Geometry check sheet. Reference: the model listing, model coordinates, mm. Face numbers are marked on the shaded views. A direction names the side the tool comes from. Round coordinates to 2 decimals unless told otherwise and drop trailing zeros. Write each loop counter-clockwise with the first axis right and the second up, starting at its lowest first coordinate (ties: lowest second). Pieces come first, ordered by that corner, then holes. Notation, with made-up numbers: M 1,-26.75 L 59,-26.75 A18 ccw 59,2.25 Z; hole C -14.5,31.5 d5. An arc over 180 degrees is marked long. Use a Markdown table: item, result.
```python
from build123d import *

# Parameters (mm, degrees)
EXTRUDE_1_DEPTH               = 9
CUT_EXTRUDE_1_DEPTH           = 30.816103032
CUT_EXTRUDE_1_DEPTH_BACK      = 30.816103032
SKETCH_2_R                    = 2.3
CUT_EXTRUDE_2_DEPTH           = 3.3
CUT_EXTRUDE_2_OTHER_WAY_DEPTH = 36.043722716
CUT_EXTRUDE_2_OTHER_WAY_TAPER = 1
CUT_EXTRUDE_3_DEPTH           = 36.043722716
CUT_EXTRUDE_3_DEPTH_BACK      = 4
CUT_EXTRUDE_4_REACH           = 46.777
CUT_EXTRUDE_4_END_RADIUS      = 10.2
SKETCH_5_R                    = 1.6
EXTRUDE_2_DEPTH               = 3
SKETCH_7_W                    = 6.2
SKETCH_7_H                    = 6
CUT_EXTRUDE_6_DEPTH           = 1
CHAMFER_3_SIZE                = 1
CUT_EXTRUDE_8_REACH           = 35.645
SKETCH_9_R                    = 2.2
CUT_EXTRUDE_9_DEPTH           = 30.816103122
CUT_EXTRUDE_START             = 5.5
SKETCH_10_R                   = 4
SKETCH_10_R_2                 = 2.2
CUT_EXTRUDE_10_DEPTH          = 5.5


with BuildPart() as part:
    # Эскиз1 → Бобышка-Вытянуть1 (new, symmetric)
    with BuildSketch(Plane(origin=(0, 0, 0), x_dir=(0, 0, -1), z_dir=(1, 0, 0))):
        with BuildLine():
            Line((-0.75, -21), (-0.75, -11.06243644))
            ThreePointArc((-0.75, -11.06243644), (-0.989654684, -10.412917388), (-1.59375, -10.074718901))
            ThreePointArc((-1.59375, -10.074718901), (0, 10.2), (1.59375, -10.074718901))
            ThreePointArc((1.59375, -10.074718901), (0.989654684, -10.412917388), (0.75, -11.06243644))
            Line((0.75, -11.06243644), (0.75, -21))
            ThreePointArc((0.75, -21), (1.042893219, -21.707106781), (1.75, -22))
            Line((1.75, -22), (6.75, -22))
            ThreePointArc((6.75, -22), (7.457106781, -21.707106781), (7.75, -21))
            Line((7.75, -21), (7.75, -13.898830886))
            ThreePointArc((7.75, -13.898830886), (8.121662204, -12.215036114), (9.167582418, -10.844142779))
            ThreePointArc((9.167582418, -10.844142779), (13.897042702, -2.917568189), (12.75462481, 6.241758242))
            ThreePointArc((12.75462481, 6.241758242), (12.953882386, 10.117431577), (16.34747687, 12))
            Line((16.34747687, 12), (17, 12))
            ThreePointArc((17, 12), (17.707106781, 12.292893219), (18, 13))
            Line((18, 13), (18, 18))
            Line((18, 18), (-18, 18))
            Line((-18, 18), (-18, 13))
            ThreePointArc((-18, 13), (-17.707106781, 12.292893219), (-17, 12))
            Line((-17, 12), (-16.34747687, 12))
            ThreePointArc((-16.34747687, 12), (-12.953882386, 10.117431577), (-12.75462481, 6.241758242))
            ThreePointArc((-12.75462481, 6.241758242), (-13.897042702, -2.917568189), (-9.167582418, -10.844142779))
            ThreePointArc((-9.167582418, -10.844142779), (-8.121662204, -12.215036114), (-7.75, -13.898830886))
            Line((-7.75, -13.898830886), (-7.75, -21))
            ThreePointArc((-7.75, -21), (-7.457106781, -21.707106781), (-6.75, -22))
            Line((-6.75, -22), (-1.75, -22))
            ThreePointArc((-1.75, -22), (-1.042893219, -21.707106781), (-0.75, -21))
        make_face()
    extrude(amount=EXTRUDE_1_DEPTH, both=True)

    # Эскиз2 → Вырез-Вытянуть1 (cut, two sides: drawn at the far end of the back side and taken through both)
    with BuildSketch(Plane.XY.offset(-CUT_EXTRUDE_1_DEPTH_BACK)):
        with BuildLine():
            ThreePointArc((-3.1, 18), (0, 14.9), (3.1, 18))
            Line((3.1, 18), (-3.1, 18))
        make_face()
        with Locations(Location((0, -16, 0), (0, 0, 66.000891847))):
            Circle(SKETCH_2_R)
    extrude(amount=CUT_EXTRUDE_1_DEPTH + CUT_EXTRUDE_1_DEPTH_BACK, mode=Mode.SUBTRACT)

    # Эскиз3 → Вырез-Вытянуть2 (cut)
    with BuildSketch(Plane(origin=(0, 0, -7.75), x_dir=(-1, 0, 0), z_dir=(0, 0, -1))):
        Polygon((-4.618802154, -16), (-2.309401077, -20), (2.309401077, -20), (4.618802154, -16), (2.309401077, -12), (-2.309401077, -12), align=None)
    extrude(amount=-CUT_EXTRUDE_2_DEPTH, mode=Mode.SUBTRACT)

    # Эскиз3 → Вырез-Вытянуть2 other way (cut)
    with BuildSketch(Plane(origin=(0, 0, -7.75), x_dir=(-1, 0, 0), z_dir=(0, 0, -1))):
        Polygon((-4.618802154, -16), (-2.309401077, -20), (2.309401077, -20), (4.618802154, -16), (2.309401077, -12), (-2.309401077, -12), align=None)
    extrude(amount=CUT_EXTRUDE_2_OTHER_WAY_DEPTH, taper=CUT_EXTRUDE_2_OTHER_WAY_TAPER, mode=Mode.SUBTRACT)

    # Эскиз4 → Вырез-Вытянуть3 (cut, two sides: drawn at the far end of the back side and taken through both)
    with BuildSketch(Plane.XY.offset(7.75).offset(-CUT_EXTRUDE_3_DEPTH_BACK)):
        with BuildLine():
            Line((-3.403687464, -13.898830886), (-0.935461573, -13.898830886))
            ThreePointArc((-0.935461573, -13.898830886), (0, -18.3), (0.935461573, -13.898830886))
            Line((0.935461573, -13.898830886), (3.403687464, -13.898830886))
            ThreePointArc((3.403687464, -13.898830886), (0, -12), (-3.403687464, -13.898830886))
        make_face()
        with BuildLine():
            ThreePointArc((0.935461573, -13.898830886), (0, -18.3), (-0.935461573, -13.898830886))
            Line((-0.935461573, -13.898830886), (-3.403687464, -13.898830886))
            ThreePointArc((-3.403687464, -13.898830886), (-1.092073748, -19.848035204), (4, -16))
            ThreePointArc((4, -16), (3.848035204, -14.907926252), (3.403687464, -13.898830886))
            Line((3.403687464, -13.898830886), (0.935461573, -13.898830886))
        make_face()
        with BuildLine():
            Line((-3.403687464, -13.898830886), (-0.935461573, -13.898830886))
            ThreePointArc((-0.935461573, -13.898830886), (0, -18.3), (0.935461573, -13.898830886))
            Line((0.935461573, -13.898830886), (3.403687464, -13.898830886))
            ThreePointArc((3.403687464, -13.898830886), (0, -12), (-3.403687464, -13.898830886))
        make_face()
        with BuildLine():
            ThreePointArc((0.935461573, -13.898830886), (0, -18.3), (-0.935461573, -13.898830886))
            Line((-0.935461573, -13.898830886), (-3.403687464, -13.898830886))
            ThreePointArc((-3.403687464, -13.898830886), (-1.092073748, -19.848035204), (4, -16))
            ThreePointArc((4, -16), (3.848035204, -14.907926252), (3.403687464, -13.898830886))
            Line((3.403687464, -13.898830886), (0.935461573, -13.898830886))
        make_face()
    extrude(amount=CUT_EXTRUDE_3_DEPTH + CUT_EXTRUDE_3_DEPTH_BACK, mode=Mode.SUBTRACT)

    # Вырез-Вытянуть4: up to this cylinder (the profile starts outside it)
    cut_extrude_4_end = Plane(origin=(0, 0, 0), z_dir=(-1, 0, 0)) * Cylinder(CUT_EXTRUDE_4_END_RADIUS, 127.454, mode=Mode.PRIVATE)
    # Эскиз5 → Вырез-Вытянуть4 (cut, up to the surface)
    with BuildSketch(Plane(origin=(0, 18, 0), x_dir=(1, 0, 0), z_dir=(0, 1, 0)), mode=Mode.PRIVATE) as cut_extrude_4_sk1:
        with Locations(Location((6.25, 0, 0), (0, 0, 270))):
            Circle(SKETCH_5_R)
    cut_extrude_4_tool1 = extrude(cut_extrude_4_sk1.sketch, amount=-CUT_EXTRUDE_4_REACH, mode=Mode.PRIVATE) - cut_extrude_4_end
    add(cut_extrude_4_tool1.solids().sort_by_distance((6.25, 18, 0))[0], mode=Mode.SUBTRACT)
    # Эскиз5 → Вырез-Вытянуть4 (cut, up to the surface)
    with BuildSketch(Plane(origin=(0, 18, 0), x_dir=(1, 0, 0), z_dir=(0, 1, 0)), mode=Mode.PRIVATE) as cut_extrude_4_sk2:
        with Locations(Location((-6.25, 0, 0), (0, 0, 270))):
            Circle(SKETCH_5_R)
    cut_extrude_4_tool2 = extrude(cut_extrude_4_sk2.sketch, amount=-CUT_EXTRUDE_4_REACH, mode=Mode.PRIVATE) - cut_extrude_4_end
    add(cut_extrude_4_tool2.solids().sort_by_distance((-6.25, 18, 0))[0], mode=Mode.SUBTRACT)

    # Эскиз6 → Бобышка-Вытянуть2 (add, symmetric)
    with BuildSketch(Plane.XY):
        with BuildLine():
            Line((-3.1, 18), (3.1, 18))
            ThreePointArc((3.1, 18), (0, 14.9), (-3.1, 18))
        make_face()
    extrude(amount=EXTRUDE_2_DEPTH, both=True)

    # Эскиз7 → Вырез-Вытянуть6 (cut)
    with BuildSketch(Plane(origin=(0, 18, 0), x_dir=(1, 0, 0), z_dir=(0, 1, 0))):
        Rectangle(SKETCH_7_W, SKETCH_7_H)
    extrude(amount=-CUT_EXTRUDE_6_DEPTH, mode=Mode.SUBTRACT)

    # Фаска3
    # the kernel refuses this chamfer: 1 mm, written as the material it adds along each edge
    with BuildSketch(Plane(origin=(3.1, 17, -3), x_dir=(0.02749587661058651, 0.9996219169112968, 0), z_dir=(0, 0, 1))) as chamfer_3_piece_1_section:
        Polygon((CHAMFER_3_SIZE * 0.999621916911, CHAMFER_3_SIZE * 0.0274958766106), (-CHAMFER_3_SIZE * 0.0274958766106, CHAMFER_3_SIZE * 0.999621916911), (0, 0), align=None)
    chamfer_3_piece_1 = extrude(amount=6, mode=Mode.PRIVATE)
    chamfer_3_piece_1 = split(chamfer_3_piece_1, bisect_by=Plane(origin=(2.769595846, 18, 0), z_dir=(0, -1, 0)), keep=Keep.TOP, mode=Mode.PRIVATE)
    add(chamfer_3_piece_1)
    with BuildSketch(Plane(origin=(-3.1, 17, 3), x_dir=(-0.02749587661058651, 0.9996219169112968, 0), z_dir=(0, 0, -1))) as chamfer_3_piece_2_section:
        Polygon((CHAMFER_3_SIZE * 0.999621916911, CHAMFER_3_SIZE * 0.0274958766106), (-CHAMFER_3_SIZE * 0.0274958766106, CHAMFER_3_SIZE * 0.999621916911), (0, 0), align=None)
    chamfer_3_piece_2 = extrude(amount=6, mode=Mode.PRIVATE)
    chamfer_3_piece_2 = split(chamfer_3_piece_2, bisect_by=Plane(origin=(-2.769595846, 18, 0), z_dir=(0, -1, 0)), keep=Keep.TOP, mode=Mode.PRIVATE)
    add(chamfer_3_piece_2)

    # Вырез-Вытянуть8: up to this plane
    cut_extrude_8_end = Plane(origin=(3.1, 18, 0), z_dir=(-0.7071067811865525, 0.7071067811865426, 0))
    # Эскиз8 → Вырез-Вытянуть8 (cut, up to the surface)
    with BuildSketch(Plane(origin=(9, 0, 0), x_dir=(0, 0, -1), z_dir=(1, 0, 0)), mode=Mode.PRIVATE) as cut_extrude_8_sk1:
        with BuildLine():
            ThreePointArc((-10.25, 18), (-6.75, 14.5), (-3.25, 18))
            Line((-3.25, 18), (-10.25, 18))
        make_face()
    cut_extrude_8_tool1 = split(extrude(cut_extrude_8_sk1.sketch, amount=-CUT_EXTRUDE_8_REACH, mode=Mode.PRIVATE), bisect_by=cut_extrude_8_end, keep=Keep.BOTH, mode=Mode.PRIVATE)
    add(cut_extrude_8_tool1.solids().sort_by_distance((9, 16.514554, 6.75))[0], mode=Mode.SUBTRACT)
    # Эскиз8 → Вырез-Вытянуть8 (cut, up to the surface)
    with BuildSketch(Plane(origin=(9, 0, 0), x_dir=(0, 0, -1), z_dir=(1, 0, 0)), mode=Mode.PRIVATE) as cut_extrude_8_sk2:
        with BuildLine():
            ThreePointArc((3.25, 18), (6.75, 14.5), (10.25, 18))
            Line((10.25, 18), (3.25, 18))
        make_face()
    cut_extrude_8_tool2 = split(extrude(cut_extrude_8_sk2.sketch, amount=-CUT_EXTRUDE_8_REACH, mode=Mode.PRIVATE), bisect_by=cut_extrude_8_end, keep=Keep.BOTH, mode=Mode.PRIVATE)
    add(cut_extrude_8_tool2.solids().sort_by_distance((9, 16.514554, -6.75))[0], mode=Mode.SUBTRACT)

    # Эскиз9 → Вырез-Вытянуть9 (cut, through all)
    with BuildSketch(Plane.XY):
        Circle(SKETCH_9_R)
    extrude(amount=-CUT_EXTRUDE_9_DEPTH, mode=Mode.SUBTRACT)

    # Эскиз10 → Вырез-Вытянуть10 (cut)
    with BuildSketch(Plane.XY.offset(-18).offset(CUT_EXTRUDE_START)):
        with Locations(Location((0, 0, 0), (0, 0, 180))):
            Circle(SKETCH_10_R)
        Circle(SKETCH_10_R_2, mode=Mode.SUBTRACT)
    extrude(amount=-CUT_EXTRUDE_10_DEPTH, mode=Mode.SUBTRACT)


solid = part.part
```
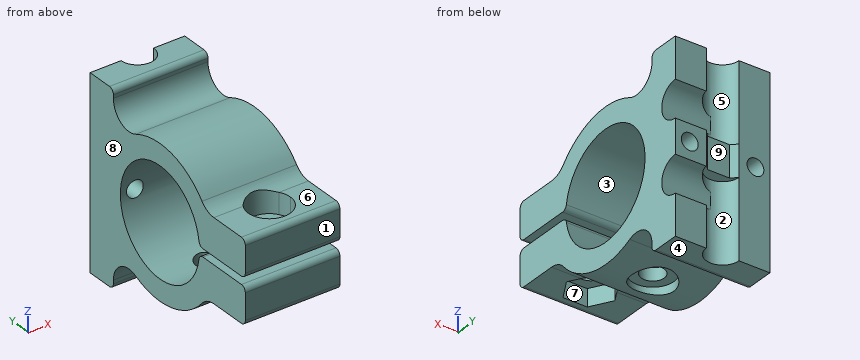
Item 1: Mould release check, pull along Y, two halves, no side actions. Record for the marked faces 1, 2, 3 and 4: +Y half, -Y half, draft (parallel to the pull), parting line (faces both ways), or undercut.
Outcome:
| item | result |
|---|---|
| face 1 | -Y half |
| face 2 | +Y half |
| face 3 | undercut |
| face 4 | draft |
Item 2: Go/stop test with flat-tipped pins: pin 1 (5 mm diameter, centred on x = -2.5, y = -18, fed in from -Z); pin 2 (1.5 mm diameter, centred on x = 1, y = 16.5, fed in from +Z); pin 3 (3 mm diameter, centred on x = -2, z = -9.5, fed in from -Y); pin 4 (10 mm diameter, centred on y = 2.5, z = -2.5, fed in from +X). Record where each tip stops, or that it passes through.
Outcome:
| item | result |
|---|---|
| pin 1 | stops at z = -7.75 |
| pin 2 | stops at z = 3 |
| pin 3 | stops at y = -12.31 |
| pin 4 | passes through |
Item 3: Cross-section at A-A, the plane z = 0. Record the cut outline in (x, y).
Outcome:
| item | result |
|---|---|
| outline | M -9,10.2 L -7.85,10.2 L -7.85,18 L -9,18 Z; M -4.65,10.2 L 4.65,10.2 L 4.65,18 L 3.1,18 L 2.1,17 L -2.1,17 L -3.1,18 L -4.65,18 Z; M 7.85,10.2 L 9,10.2 L 9,18 L 7.85,18 Z |
Item 4: Cross-section at D-D, the plane y = 4.5. Record the cut outline in (x, z), and give its area (3 significant figures).
Outcome:
| item | result |
|---|---|
| outline | M -9,-13.47 L 9,-13.47 L 9,-9.15 L -9,-9.15 Z; M -9,9.15 L 9,9.15 L 9,13.47 L -9,13.47 Z |
| area | 155 mm2 |
Item 5: Cross-section at B-B, the plane y = 0. Record the cut outline in (x, z), and give its area (3 significant figures).
Outcome:
| item | result |
|---|---|
| outline | M -9,-14.2 L -4,-14.2 L -4,-12.5 L -2.2,-12.5 L -2.2,-10.2 L -9,-10.2 Z; M -9,10.2 L 9,10.2 L 9,14.2 L -9,14.2 Z; M 2.2,-12.5 L 4,-12.5 L 4,-14.2 L 9,-14.2 L 9,-10.2 L 2.2,-10.2 Z |
| area | 120 mm2 |
Item 6: Material ranges on line 1 along Z through (x, y) = (-6.25, 13.25); line 2 along X through (y, z) = (-16, 6.6); line 3 along X through (y, z) = (-16, 2), recorded low to high. Write a range as from..to.
Outcome:
| item | result |
|---|---|
| line 1 | z = -18..-1.6, 1.6..18 |
| line 2 | x = -9..-4, 4..9 |
| line 3 | x = -9..-2.3, 2.3..9 |
Item 7: Access from +Z, -Z, +X, -X, +Y, -Y to the whole of each face (thin tool, end or side, straight path). Record for the marked faces 5, 6, 7, 8 and 9.
Outcome:
| item | result |
|---|---|
| face 5 | +Z, +Y |
| face 6 | +Z, +X, -X, -Y |
| face 7 | -Z |
| face 8 | +Z, -Z, -X, +Y, -Y |
| face 9 | +Z, -Z, +Y |
